CAD build for the part. Positions are in the model's coordinates, mm. Round coordinates to 2 decimals unless told otherwise and drop trailing zeros. Write each loop counter-clockwise with the first axis right and the second up, starting at its lowest first coordinate (ties: lowest second). Pieces come first, ordered by that corner, then holes. Notation, with made-up numbers: (59, 3.25) - (85, 3.25) arc R22 ccw to (85, 16.25) - close; hole circle Ø1 at (84.25, 19). An arc over 180 degrees is marked (long way). Answer in a Markdown table with one row per item.
```python
from build123d import *

# Parameters (mm, degrees)
SKETCH1_R           = 7
SKETCH1_R_2         = 2.75
BOSS_EXTRUDE1_DEPTH = 34
CHAMFER1_SIZE       = 0.5
CHAMFER2_SIZE       = 0.5


with BuildPart() as part:
    # Sketch1 → Boss-Extrude1 (new, symmetric)
    with BuildSketch(Plane(origin=(0, 0, 0), x_dir=(0, 1, 0), z_dir=(0, 0, 1))):
        with Locations(Location((0, 0, 0), (0, 0, 270))):
            Circle(SKETCH1_R)
        with Locations(Location((0, 0, 0), (0, 0, 270))):
            Circle(SKETCH1_R_2, mode=Mode.SUBTRACT)
    extrude(amount=BOSS_EXTRUDE1_DEPTH, both=True)

    # Chamfer1
    chamfer1_edges = [part.edges().sort_by_distance(p)[0] for p in [
        (-2.75, 0, -34),
        (-2.75, 0, 34),
    ]]
    chamfer(chamfer1_edges, length=CHAMFER1_SIZE)

    # Chamfer2
    chamfer2_edges = [part.edges().sort_by_distance(p)[0] for p in [
        (-7, 0, -34),
        (-7, 0, 34),
    ]]
    chamfer(chamfer2_edges, length=CHAMFER2_SIZE)


solid = part.part
```
Q1. Saw through at C-C on z = 27.5. List the corners of the cut face in (x, y).
Computed:
| item | result |
|---|---|
| outline | circle Ø14 at (0, 0); hole circle Ø5.5 at (0, 0) |
Q2. Pull direction X, two halves, no side cores. Call faces 1 (the cylindrical face through (-1.517, -6.834, 0.469)), 2 (the flat face through (-2, 3, 34)), 3 (the cylindrical face through (-0.596, -2.685, -0.469)): released by +X, released by -X, zero draft, split by the parting line, or undercut.
Computed:
| item | result |
|---|---|
| face 1 | split by the parting line |
| face 2 | zero draft |
| face 3 | undercut |
Q3. Drill centre lines: line 1 (Y direction, x = 0, z = -4); line 2 (Y direction, x = -1.5, z = -13); line 3 (X direction, y = 0.75, z = -5.5). Where is each one in solid material? Low to high.
Computed:
| item | result |
|---|---|
| line 1 | y = -7 to -2.75, 2.75 to 7 |
| line 2 | y = -6.84 to -2.3, 2.3 to 6.84 |
| line 3 | x = -6.96 to -2.65, 2.65 to 6.96 |
Q4. Saw through at A-A on y = 0. List the corners of the cut face in (x, z).
Computed:
| item | result |
|---|---|
| outline | (-7, -33.5) - (-6.5, -34) - (-3.25, -34) - (-2.75, -33.5) - (-2.75, 33.5) - (-3.25, 34) - (-6.5, 34) - (-7, 33.5) - close; (2.75, -33.5) - (3.25, -34) - (6.5, -34) - (7, -33.5) - (7, 33.5) - (6.5, 34) - (3.25, 34) - (2.75, 33.5) - close |
Q5. Flat gauge pins, fed straight in: pin 1 (5 mm diameter, centred on x = 5.5, z = 4, fed in from +Y); pin 2 (3 mm diameter, centred on y = 3, z = 16, fed in from +X); pin 3 (4 mm diameter, centred on y = -2.5, z = 12, fed in from +X). Where does each tip first touch, or does it go through?
Computed:
| item | result |
|---|---|
| pin 1 | stops at y = 6.32 |
| pin 2 | stops at x = 6.84 |
| pin 3 | stops at x = 6.98 |
